Read the model definition and answer for the solid it produces. Units are mm, in the model's axes. A direction names the side the tool comes from. Round coordinates to 2 decimals unless told otherwise and drop trailing zeros. Loops run counter-clockwise (first coordinate to the right, second up) from the corner with the lowest first, then second, coordinate; pieces in that order, holes last. Notation, with made-up numbers: M 40,39.25 L 94,39.25 A17 ccw 94,63.25 Z; hole C -0.75,-6 d3. An arc over 180 degrees is marked long. Answer as CSV lines item,"result".
```python
from build123d import *

# Parameters (mm, degrees)
HEAD_DEPTH     = 10
SHANK_SKETCH_R = 6.096
SHANK_DEPTH    = 101.6
SKETCH6_R      = 8.001
HEAD_CUT_DEPTH = 1.5
FILLET1_R      = 2
FILLET2_R      = 0.5
THREAD_END_W   = 88.9
THREAD_END_H   = 0.05


with BuildPart() as part:
    # Head Sketch → Head (new body)
    with BuildSketch(Plane.XY):
        Polygon((0, 10.558581723), (9.144, 5.279290861), (9.144, -5.279290861), (0, -10.558581723), (-9.144, -5.279290861), (-9.144, 5.279290861), align=None)
    extrude(amount=HEAD_DEPTH)

    # Shank Sketch → Shank (add)
    with BuildSketch(Plane.XY):
        Circle(SHANK_SKETCH_R)
    extrude(amount=-SHANK_DEPTH)

    # Sketch3 → Flange (revolve)
    with BuildSketch(Plane(origin=(0, 0, 0), x_dir=(-1, 0, 0), z_dir=(0, 1, 0)), mode=Mode.PRIVATE) as flange_sk:
        with BuildLine():
            Line((-10.668, 0), (0, 0))
            Line((0, 0), (0, 3.81))
            ThreePointArc((0, 3.81), (-5.643297007, 3.079227926), (-10.91431477, 0.935119563))
            ThreePointArc((-10.91431477, 0.935119563), (-11.151507901, 0.372641807), (-10.668, 0))
        make_face()
    revolve(flange_sk.sketch.rotate(Axis((0, 0, 0), (0, 0, 1)), 30), axis=Axis((0, 0, 0), (0, 0, 1)))

    # Sketch5 → Head Trim (revolve, cut)
    with BuildSketch(Plane(origin=(0, 0, 0), x_dir=(0, 0, -1), z_dir=(1, 0, 0)), mode=Mode.PRIVATE) as head_trim_sk:
        with BuildLine():
            Line((-10, -8.558581723), (-10, -10.558581723))
            Line((-10, -10.558581723), (-8, -10.558581723))
            ThreePointArc((-8, -10.558581723), (-9.414213562, -9.972795285), (-10, -8.558581723))
        make_face()
    revolve(head_trim_sk.sketch.rotate(Axis((0, 0, 15.085599173), (0, 0, -1)), 90), axis=Axis((0, 0, 15.085599173), (0, 0, -1)), mode=Mode.SUBTRACT)

    # Sketch6 → Head Cut (cut)
    with BuildSketch(Plane.XY.offset(10)):
        Circle(SKETCH6_R)
    extrude(amount=-HEAD_CUT_DEPTH, mode=Mode.SUBTRACT)

    # Fillet1
    # the kernel refuses this fillet: 2 mm, written as the material it adds along each edge
    with BuildSketch(Plane(origin=(0, 0, 8.5), x_dir=(1, 0, 0), z_dir=(0, -1, 0))) as fillet1_piece_1:
        with BuildLine():
            CenterArc((6.064508327, 2), FILLET1_R, 270, 75.522487814)
            Line((6.064508327, 0), (6.064508327, -0.04))
            Line((6.064508327, -0.04), (8.001, -0.04))
            Line((8.001, -0.04), (8.041, 0))
            ThreePointArc((8.041, 0), (8.041, 0.75), (8.039729833, 1.49))
            Line((8.039729833, 1.49), (8.001, 1.5))
        make_face()
    revolve(axis=Axis((0, 0, 8.5), (0, 0, 1)))

    # Fillet2
    fillet2_edges = [part.edges().sort_by_distance(p)[0] for p in [
        (-6.096, 0, 0),
    ]]
    fillet(fillet2_edges, radius=FILLET2_R)

    # Thread End → Thread Cut (revolve, cut)
    with BuildSketch(Plane(origin=(0, 0, 0), x_dir=(0, 0, -1), z_dir=(1, 0, 0)), mode=Mode.PRIVATE) as thread_cut_sk:
        with Locations((57.15, 6.071)):
            Rectangle(THREAD_END_W, THREAD_END_H)
    revolve(thread_cut_sk.sketch.rotate(Axis((0, 0, -21.551935625), (0, 0, -1)), 90), axis=Axis((0, 0, -21.551935625), (0, 0, -1)), mode=Mode.SUBTRACT)


solid = part.part
```
1) Find section A-A, the plane z = -27.5. Give the vertices of the cut face in (x, y), then the cut area to 3 significant figures.
Evaluation:
outline,"C 0,0 d12.09"
area,"115 mm^2"
2) Straight lines are drawn through the part: line 1 (Z direction, x = -5.5, y = -6.25); line 2 (Z direction, x = 1.5, y = -2.5); line 3 (X direction, y = 2.25, z = 2). For each, find the intervals that lie inside material, in ascending order.
Evaluation:
line 1,"z = 0 to 10"
line 2,"z = -101.6 to 8.5"
line 3,"x = -9.14 to 9.14"
3) Find section B-B, the plane z = -6. Give the vertices of the cut face in (x, y), then the cut area to 3 significant figures.
Evaluation:
outline,"C 0,0 d12.19"
area,"117 mm^2"
4) Determine the mould class of faces 1 (the flat face through (0, 0, -101.6)), 2 (the cylindrical face through (-0.794, 6.044, -6.515)), 3 (the flat face through (0, 0, 8.5)), 4 (the flat face through (4.64, -7.88, 5.46)) for opening direction X: released by +X, released by -X, zero draft, split by the parting line, or undercut.
Evaluation:
face 1,"zero draft"
face 2,"split by the parting line"
face 3,"undercut"
face 4,"released by +X"
5) A tool of negligible diameter and unlimited length cuts with its end or side. For faces 5 (the flat face through (4.508, 7.956, 5.461)), 6 (the flat face through (-4.508, -7.956, 5.461)), 7 (the flat face through (2, 7, 0)), from which of +Z, -Z, +X, -X, +Y, -Y can it reach the whole face along a straight path? Write none if from no direction.
Evaluation:
face 5,"+Z, +X, +Y"
face 6,"+Z, -X, -Y"
face 7,"-Z"
6) Each of these flat-tipped pins is pushed along its axis until it touches: P1, Ø2, axis at y = -3.5, z = -70, coming from the +X side; P2, Ø6, axis at y = 3, z = -75, coming from the +X side; P3, Ø8, axis at x = -2.5, z = -75.5, coming from the -Y side. Where does it stop, or does it pass through?
Evaluation:
P1,"stops at x = 5.5"
P2,"stops at x = 6.05"
P3,"stops at y = -6.05"
